Source: CAD feature listing. Evaluate the final solid. Frame: model axes, mm. A direction names the side the tool comes from. Coordinates: 2 decimals unless noted, no trailing zeros. Order: outer loops, then holes, each group sorted by start corner. A loop starts at its lowest first (then second) coordinate and runs counter-clockwise, first axis right, second up.
```python
from build123d import *

# Parameters (mm, degrees)
SKETCH1_W           = 177.8
SKETCH1_H           = 101.6
BOSS_EXTRUDE1_DEPTH = 6.35
SKETCH2_R           = 14.859
CUT_EXTRUDE1_DEPTH  = 6.35
SKETCH3_R           = 25.4
CUT_EXTRUDE2_DEPTH  = 2.5654
SKETCH4_R           = 4.7625
CUT_EXTRUDE3_DEPTH  = 20.3454
CIRPATTERN1_COUNT   = 8


with BuildPart() as part:
    # Sketch1 → Boss-Extrude1 (new body)
    with BuildSketch(Plane(origin=(0, 0, 0), x_dir=(1, 0, 0), z_dir=(0, 1, 0))):
        Rectangle(SKETCH1_W, SKETCH1_H)
    extrude(amount=BOSS_EXTRUDE1_DEPTH)

    # Sketch2 → Cut-Extrude1 (cut)
    with BuildSketch(Plane(origin=(0, 6.35, 0), x_dir=(1, 0, 0), z_dir=(0, 1, 0))):
        with Locations(Location((0, 0, 0), (0, 0, 270))):
            Circle(SKETCH2_R)
    extrude(amount=-CUT_EXTRUDE1_DEPTH, mode=Mode.SUBTRACT)

    # Sketch3 → Cut-Extrude2 (cut)
    with BuildSketch(Plane(origin=(0, 6.35, 0), x_dir=(1, 0, 0), z_dir=(0, 1, 0))):
        with Locations(Location((0, 0, 0), (0, 0, 270))):
            Circle(SKETCH3_R)
    extrude(amount=-CUT_EXTRUDE2_DEPTH, mode=Mode.SUBTRACT)

    # Sketch4 → Cut-Extrude3 (cut)
    with BuildSketch(Plane(origin=(0, 6.35, 0), x_dir=(1, 0, 0), z_dir=(0, 1, 0))):
        with Locations(Location((1.623422677, 41.37015957, 0), (0, 0, 270))):
            Circle(SKETCH4_R)
    cut_extrude3 = extrude(amount=-CUT_EXTRUDE3_DEPTH, mode=Mode.SUBTRACT)

    # CirPattern1: Cut-Extrude3 ×8 about axis
    cirpattern1_axis = Axis((0, 0, 0), (0, 1, 0))
    for i in range(1, CIRPATTERN1_COUNT):
        add(cut_extrude3.rotate(cirpattern1_axis, i * 360 / CIRPATTERN1_COUNT), mode=Mode.SUBTRACT)


solid = part.part
```
Q1. Section query C-C on x = -17. Output: boundary loops of the cut face in (y, z), plus the area to 3 significant figures.
Solutions:
outline: (0, -50.8) - (6.35, -50.8) - (6.35, -18.87) - (3.78, -18.87) - (3.78, 18.87) - (6.35, 18.87) - (6.35, 50.8) - (0, 50.8) - close
area: 548 mm2
Q2. Pull-direction query (Z, two-part tool) for faces 3 (the flat face through (-1, 3, -50.8)), 4 (the flat face through (-21, 0, -1)), 5 (the flat face through (-11, 3.785, 11)); classes: pulls with the +Z half, pulls with the -Z half, needs draft (parallel to the pull), parting line crosses it, or undercut.
Solutions:
face 3: pulls with the -Z half
face 4: needs draft
face 5: undercut
Q3. Material intervals for line 1 along Z through (x, y) = (-41, 5.75); line 2 along X through (y, z) = (1, 6); line 3 along Z through (x, y) = (28.5, 2.5), sorted ascending.
Solutions:
line 1: z = -50.8 to -6.37, 3.12 to 50.8
line 2: x = -88.9 to -13.59, 13.59 to 39.49, 43.25 to 88.9
line 3: z = -50.8 to -32.47, -23.74 to 25.65, 35.15 to 50.8
Q4. Section query B-B on z = 44. Output: boundary loops of the cut face in (x, y).
Solutions:
outline: (-88.9, 0) - (-5.59, 0) - (-5.59, 6.35) - (-88.9, 6.35) - close; (2.35, 0) - (88.9, 0) - (88.9, 6.35) - (2.35, 6.35) - close
Q5. Section query D-D on z = 10. Output: boundary loops of the cut face in (x, y).
Solutions:
outline: (-88.9, 0) - (-10.99, 0) - (-10.99, 3.78) - (-23.35, 3.78) - (-23.35, 6.35) - (-88.9, 6.35) - close; (10.99, 0) - (88.9, 0) - (88.9, 6.35) - (23.35, 6.35) - (23.35, 3.78) - (10.99, 3.78) - close
Q6. Set-up query: faces 1 (the cylindrical face through (-15.456, 5.085, -20.157)), 2 (the cylindrical face through (-5.691, 1.919, 13.726)). Return all of +Z, -Z, +X, -X, +Y, -Y with unobstructed straight access to the full face (end or side cutting, diameter ignored); none if empty.
Solutions:
face 1: +Y
face 2: +Y, -Y
Q7. Section query A-A on y = 2.75. Give the number of separate pieces and of enclosed holes in the cut face, plus the area to 3 significant figures.
Solutions:
separate pieces: 1
enclosed holes: 9
area: 16,800 mm2
